Build history of the part. All positions in model axes, mm. A direction names the side the tool comes from. Round coordinates to 2 decimals unless told otherwise and drop trailing zeros. Write each loop counter-clockwise with the first axis right and the second up, starting at its lowest first coordinate (ties: lowest second). Pieces come first, ordered by that corner, then holes. Notation, with made-up numbers: M 39.5,-2.5 L 59.5,-2.5 A21 cw 59.5,22.5 Z; hole C 72,51 d7. An arc over 180 degrees is marked long. Write item = value, one per line.
from build123d import *

# Parameters (mm, degrees)
BOSS_EXTRUDE1_DEPTH = 23
CUT_EXTRUDE1_DEPTH  = 24
SKETCH3_W           = 15
SKETCH3_H           = 12.914285714
CUT_EXTRUDE2_DEPTH  = 39.3
CUT_EXTRUDE4_DEPTH  = 3.285714286
SKETCH4_W           = 15
SKETCH4_H           = 1.142857143
CUT_EXTRUDE3_DEPTH  = 39.3
SKETCH_1_R          = 8.1
CUT_EXTRUDE_1_DEPTH = 2.285714
BOSS_EXTRUDE3_START = -2.285714
SKETCH7_R           = 2.5
BOSS_EXTRUDE3_DEPTH = 2.285714
EXTRUDE_START       = -20.714286
SKETCH7_2_R         = 2.5
EXTRUDE_1_DEPTH     = 2.285714
CHAMFER1_SIZE       = 0.5


with BuildPart() as part:
    # Sketch1 → Boss-Extrude1 (new body)
    with BuildSketch(Plane.XY):
        with BuildLine():
            Line((-15.35, 7.6), (15.35, 7.6))
            ThreePointArc((15.35, 7.6), (22.95, 0), (15.35, -7.6))
            Line((15.35, -7.6), (-15.35, -7.6))
            ThreePointArc((-15.35, -7.6), (-22.95, 0), (-15.35, 7.6))
        make_face()
    extrude(amount=-BOSS_EXTRUDE1_DEPTH)

    # Sketch2 → Cut-Extrude1 (cut, through all)
    with BuildSketch(Plane.XY):
        with BuildLine():
            Line((-8.239692572, 2.683938949), (15.35, -5))
            Line((15.35, -5), (15.35, -7.6))
            ThreePointArc((15.35, -7.6), (22.95, 0), (15.35, 7.6))
            Line((15.35, 7.6), (-15.35, 7.6))
            ThreePointArc((-15.35, 7.6), (-11.027844057, 6.251317302), (-8.239692572, 2.683938949))
        make_face()
    extrude(amount=-CUT_EXTRUDE1_DEPTH, mode=Mode.SUBTRACT)

    # Sketch3 → Cut-Extrude2 (cut, through all)
    with BuildSketch(Plane(origin=(15.35, 0, 0), x_dir=(0, 0, -1), z_dir=(1, 0, 0))):
        with Locations((11.5, 1.142857143)):
            Rectangle(SKETCH3_W, SKETCH3_H)
    extrude(amount=-CUT_EXTRUDE2_DEPTH, mode=Mode.SUBTRACT)

    # Sketch5 → Cut-Extrude4 (cut, through all)
    with BuildSketch(Plane(origin=(0, -5.314285714, 0), x_dir=(1, 0, 0), z_dir=(0, 1, 0))):
        with BuildLine():
            Line((9.85, 15), (9.85, 8))
            ThreePointArc((9.85, 8), (7.85, 6), (5.85, 8))
            Line((5.85, 8), (5.85, 15))
            ThreePointArc((5.85, 15), (7.85, 17), (9.85, 15))
        make_face()
        with BuildLine():
            Line((-0.15, 15), (-0.15, 8))
            ThreePointArc((-0.15, 8), (-2.15, 6), (-4.15, 8))
            Line((-4.15, 8), (-4.15, 15))
            ThreePointArc((-4.15, 15), (-2.15, 17), (-0.15, 15))
        make_face()
    extrude(amount=-CUT_EXTRUDE4_DEPTH, mode=Mode.SUBTRACT)

    # Sketch4 → Cut-Extrude3 (cut, through all)
    with BuildSketch(Plane(origin=(15.35, 0, 0), x_dir=(0, 0, -1), z_dir=(1, 0, 0))):
        with Locations((11.5, -7.028571429)):
            Rectangle(SKETCH4_W, SKETCH4_H)
    extrude(amount=-CUT_EXTRUDE3_DEPTH, mode=Mode.SUBTRACT)

    # Sketch 1 → Cut-Extrude 1 (cut)
    with BuildSketch(Plane.XY):
        with Locations((-15.35, 0)):
            Circle(SKETCH_1_R)
    cut_extrude_1 = extrude(amount=-CUT_EXTRUDE_1_DEPTH, mode=Mode.SUBTRACT)

    # Sketch7 → Boss-Extrude3 (add)
    with BuildSketch(Plane.XY.offset(BOSS_EXTRUDE3_START)):
        with Locations((-15.35, 0)):
            Circle(SKETCH7_R)
    extrude(amount=BOSS_EXTRUDE3_DEPTH)

    # Mirror 1: Cut-Extrude 1 across plane
    add(cut_extrude_1.mirror(Plane.XY.offset(-11.5)), mode=Mode.SUBTRACT)

    # Sketch7_2 → Extrude 1 (add)
    with BuildSketch(Plane.XY.offset(EXTRUDE_START)):
        with Locations((-15.35, 0)):
            Circle(SKETCH7_2_R)
    extrude(amount=-EXTRUDE_1_DEPTH)

    # Chamfer1
    chamfer1_edges = [part.edges().sort_by_distance(p)[0] for p in [
        (7.85, -5.314285714, -17),
        (5.85, -5.314285714, -11.5),
        (7.85, -5.314285714, -6),
        (9.85, -5.314285714, -11.5),
        (-2.15, -5.314285714, -17),
        (-4.15, -5.314285714, -11.5),
        (-2.15, -5.314285714, -6),
        (-0.15, -5.314285714, -11.5),
    ]]
    chamfer(chamfer1_edges, length=CHAMFER1_SIZE)


solid = part.part
1. Mould opens along Z. For faces 1 (the face through (7.897, -5.679, -5.865)), 2 (the face through (-6, -5.314, -11)), 3 (the face through (0, -7.6, -2)), 4 (the face through (-13, 2, -2.286)) say: pulls with the +Z half, pulls with the -Z half, needs draft (parallel to the pull), parting line crosses it, or undercut.
Responses:
face_1 = undercut
face_2 = undercut
face_3 = needs draft
face_4 = pulls with the +Z half
2. Band-saw the part on B-B (x = -2.15). List the corners of the cut face in (y, z).
Responses:
outline = M -7.6,-23 L 0.7,-23 L 0.7,-19 L -5.31,-19 L -5.31,-17.5 L -5.81,-17 L -6.46,-17 L -6.46,-19 L -7.6,-19 Z; M -7.6,-4 L -6.46,-4 L -6.46,-6 L -5.81,-6 L -5.31,-5.5 L -5.31,-4 L 0.7,-4 L 0.7,0 L -7.6,0 Z
3. Band-saw the part on A-A (y = 5.5). List the corners of the cut face in (x, z) (3 decimals), plus the area to 3 significant figures.
Responses:
outline = M -20.595,-20.714 L -10.105,-20.714 L -10.105,-19 L -20.595,-19 Z; M -20.595,-4 L -10.105,-4 L -10.105,-2.286 L -20.595,-2.286 Z
area = 36.0 mm²
4. Flat gauge pins, fed straight in: pin 1 (5 mm diameter, centred on x = 5, z = -8, fed in from +Y); pin 2 (4.5 mm diameter, centred on x = -7, z = -13, fed in from -Y); pin 3 (0.5 mm diameter, centred on y = -6, z = -11.5, fed in from -X). Where does each tip first touch, or does it go through?
Responses:
pin_1 = -5.31
pin_2 = -6.46
pin_3 = -20.32
5. Band-saw the part on D-D (y = 0.75). List the corners of the cut face in (x, z).
Responses:
outline = M -22.91,-20.71 L -17.73,-20.71 L -17.73,-23 L -12.97,-23 L -12.97,-20.71 L -7.28,-20.71 L -7.28,-23 L -2.3,-23 L -2.3,-19 L -22.91,-19 Z; M -22.91,-4 L -2.3,-4 L -2.3,0 L -7.28,0 L -7.28,-2.29 L -12.97,-2.29 L -12.97,0 L -17.73,0 L -17.73,-2.29 L -22.91,-2.29 Z
6. Band-saw the part on C-C (x = 7.85). List the corners of the cut face in (y, z), plus the area to 3 significant figures.
Responses:
outline = M -7.6,-23 L -2.56,-23 L -2.56,-19 L -5.31,-19 L -5.31,-17.5 L -5.81,-17 L -6.46,-17 L -6.46,-19 L -7.6,-19 Z; M -7.6,-4 L -6.46,-4 L -6.46,-6 L -5.81,-6 L -5.31,-5.5 L -5.31,-4 L -2.56,-4 L -2.56,0 L -7.6,0 Z
area = 44.7 mm²
7. Probe probe 1 along Z at (x, y) = (9, -4.25); probe 2 along Z at (x, y) = (-9, -4.5); probe 3 along Y at (x, z) = (-18, -10.5). List the from-to ranges inside material, lowest first.
Responses:
probe_1 = -23 to -19, -4 to 0
probe_2 = -20.71 to -19, -4 to -2.29
probe_3 = -6.46 to -5.31
8. Tool access for faces 5 (the face through (-6, -6.457, -11)), 6 (the face through (7.9, -6.1, -6)), 7 (the face through (-2.103, -5.679, -5.865)), 8 (the face through (-12.965, 0.751, -1.159)): list every direction of +Z, -Z, +X, -X, +Y, -Y with a clear straight run to the whole face (end or side of a thin tool).
Responses:
face_5 = +X, -X, -Y
face_6 = +Y, -Y
face_7 = +Y
face_8 = +Z
